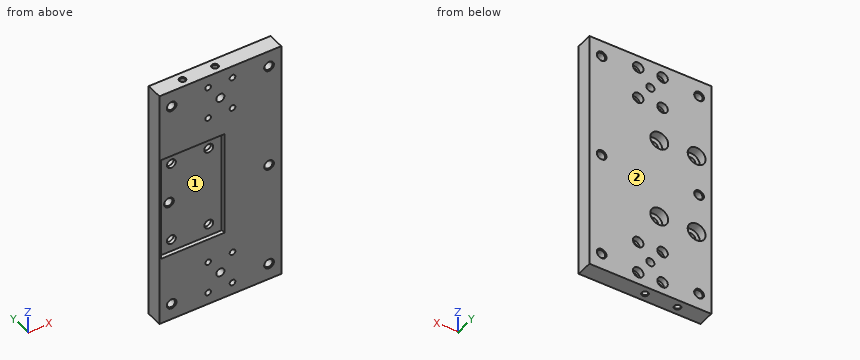
from build123d import *

# Parameters (mm, degrees)
EXTRUDE_1_DEPTH             = 75
EXTRUDE_1_DEPTH_BACK        = 75
SKETCH_1_W                  = 75
SKETCH_1_H                  = 10
SKETCH_2_W                  = 2.5
SKETCH_2_H                  = 10
SKETCH_3_W                  = 2.5
SKETCH_3_H                  = 10
PATTERN_LINEAR_2_COUNT      = 2
PATTERN_LINEAR_2_PITCH      = 23
PATTERN_LINEAR_2_COUNT_DIR2 = 2
PATTERN_LINEAR_2_PITCH_DIR2 = 50
SKETCH_15_W                 = 39
SKETCH_15_H                 = 65
CUT_EXTRUDE_1_DEPTH         = 32.5


with BuildPart() as part:
    # Sketch 1 → Extrude 1 (new, two sides: drawn at the far end of the back side and taken through both)
    with BuildSketch(Plane.XY.offset(-EXTRUDE_1_DEPTH_BACK)):
        with Locations((0, 5)):
            Rectangle(SKETCH_1_W, SKETCH_1_H)
    extrude(amount=EXTRUDE_1_DEPTH + EXTRUDE_1_DEPTH_BACK)

    # Sketch 2 → Cut-Revolve 1 (revolve, cut)
    with BuildSketch(Plane.XY.offset(57.5), mode=Mode.PRIVATE) as cut_revolve_1_sk:
        with Locations((-1.25, 5)):
            Rectangle(SKETCH_2_W, SKETCH_2_H)
    revolve(cut_revolve_1_sk.sketch.rotate(Axis((0, 10, 57.5), (0, -1, 0)), 90), axis=Axis((0, 10, 57.5), (0, -1, 0)), mode=Mode.SUBTRACT)

    # Sketch 3 → Cut-Revolve 2 (revolve, cut)
    with BuildSketch(Plane.XY.offset(-57.5), mode=Mode.PRIVATE) as cut_revolve_2_sk:
        with Locations((-1.25, 5)):
            Rectangle(SKETCH_3_W, SKETCH_3_H)
    revolve(cut_revolve_2_sk.sketch.rotate(Axis((0, 10, -57.5), (0, -1, 0)), 90), axis=Axis((0, 10, -57.5), (0, -1, 0)), mode=Mode.SUBTRACT)

    # Sketch 4 → Cut-Revolve 3 (revolve, cut)
    with BuildSketch(Plane.XY.offset(67.5), mode=Mode.PRIVATE) as cut_revolve_3_sk:
        Polygon((-7.5, 0), (-9.25, 0), (-9.25, 6.5), (-10.75, 6.5), (-10.75, 10), (-7.5, 10), align=None)
    revolve(cut_revolve_3_sk.sketch.rotate(Axis((-7.5, 10, 67.5), (0, -1, 0)), 90), axis=Axis((-7.5, 10, 67.5), (0, -1, 0)), mode=Mode.SUBTRACT)

    # Sketch 6 → Cut-Revolve 4 (revolve, cut)
    with BuildSketch(Plane.XY.offset(-47.5), mode=Mode.PRIVATE) as cut_revolve_4_sk:
        Polygon((7.5, 0), (5.75, 0), (5.75, 6.5), (4.25, 6.5), (4.25, 10), (7.5, 10), align=None)
    revolve(cut_revolve_4_sk.sketch.rotate(Axis((7.5, 10, -47.5), (0, -1, 0)), 90), axis=Axis((7.5, 10, -47.5), (0, -1, 0)), mode=Mode.SUBTRACT)

    # Sketch 7 → Cut-Revolve 5 (revolve, cut)
    with BuildSketch(Plane.XY.offset(-47.5), mode=Mode.PRIVATE) as cut_revolve_5_sk:
        Polygon((-7.5, 0), (-9.25, 0), (-9.25, 6.5), (-10.75, 6.5), (-10.75, 10), (-7.5, 10), align=None)
    revolve(cut_revolve_5_sk.sketch.rotate(Axis((-7.5, 10, -47.5), (0, -1, 0)), 90), axis=Axis((-7.5, 10, -47.5), (0, -1, 0)), mode=Mode.SUBTRACT)

    # Sketch 8 → Cut-Revolve 6 (revolve, cut)
    with BuildSketch(Plane.XY.offset(-67.5), mode=Mode.PRIVATE) as cut_revolve_6_sk:
        Polygon((7.5, 0), (5.75, 0), (5.75, 6.5), (4.25, 6.5), (4.25, 10), (7.5, 10), align=None)
    revolve(cut_revolve_6_sk.sketch.rotate(Axis((7.5, 10, -67.5), (0, -1, 0)), 90), axis=Axis((7.5, 10, -67.5), (0, -1, 0)), mode=Mode.SUBTRACT)

    # Sketch 9 → Cut-Revolve 7 (revolve, cut)
    with BuildSketch(Plane.XY.offset(-67.5), mode=Mode.PRIVATE) as cut_revolve_7_sk:
        Polygon((-7.5, 0), (-9.25, 0), (-9.25, 6.5), (-10.75, 6.5), (-10.75, 10), (-7.5, 10), align=None)
    revolve(cut_revolve_7_sk.sketch.rotate(Axis((-7.5, 10, -67.5), (0, -1, 0)), 90), axis=Axis((-7.5, 10, -67.5), (0, -1, 0)), mode=Mode.SUBTRACT)

    # Sketch 10 → Cut-Revolve 8 (revolve, cut)
    with BuildSketch(Plane.XY.offset(47.5), mode=Mode.PRIVATE) as cut_revolve_8_sk:
        Polygon((7.5, 0), (5.75, 0), (5.75, 6.5), (4.25, 6.5), (4.25, 10), (7.5, 10), align=None)
    revolve(cut_revolve_8_sk.sketch.rotate(Axis((7.5, 10, 47.5), (0, -1, 0)), 90), axis=Axis((7.5, 10, 47.5), (0, -1, 0)), mode=Mode.SUBTRACT)

    # Sketch 11 → Cut-Revolve 9 (revolve, cut)
    with BuildSketch(Plane.XY.offset(47.5), mode=Mode.PRIVATE) as cut_revolve_9_sk:
        Polygon((-7.5, 0), (-9.25, 0), (-9.25, 6.5), (-10.75, 6.5), (-10.75, 10), (-7.5, 10), align=None)
    revolve(cut_revolve_9_sk.sketch.rotate(Axis((-7.5, 10, 47.5), (0, -1, 0)), 90), axis=Axis((-7.5, 10, 47.5), (0, -1, 0)), mode=Mode.SUBTRACT)

    # Sketch 12 → Cut-Revolve 10 (revolve, cut)
    with BuildSketch(Plane.XY.offset(67.5), mode=Mode.PRIVATE) as cut_revolve_10_sk:
        Polygon((7.5, 0), (5.75, 0), (5.75, 6.5), (4.25, 6.5), (4.25, 10), (7.5, 10), align=None)
    revolve(cut_revolve_10_sk.sketch.rotate(Axis((7.5, 10, 67.5), (0, -1, 0)), 90), axis=Axis((7.5, 10, 67.5), (0, -1, 0)), mode=Mode.SUBTRACT)

    # Sketch 13 → Cut-Revolve 11 (revolve, cut)
    with BuildSketch(Plane(origin=(-28.5, 0, 0), x_dir=(0, 0, -1), z_dir=(1, 0, 0)), mode=Mode.PRIVATE) as cut_revolve_11_sk:
        Polygon((-25, 0), (-27.75, 0), (-27.75, 4.6), (-30.5, 4.6), (-30.5, 10), (-25, 10), align=None)
    cut_revolve_11 = revolve(cut_revolve_11_sk.sketch.rotate(Axis((-28.5, 10, 25), (0, -1, 0)), 180), axis=Axis((-28.5, 10, 25), (0, -1, 0)), mode=Mode.SUBTRACT)

    # Pattern Linear 2: Cut-Revolve 11 2 × 2
    with Locations(*[(i * PATTERN_LINEAR_2_PITCH, 0, -j * PATTERN_LINEAR_2_PITCH_DIR2) for i in range(PATTERN_LINEAR_2_COUNT) for j in range(PATTERN_LINEAR_2_COUNT_DIR2) if (i, j) != (0, 0)]):
        add(cut_revolve_11, mode=Mode.SUBTRACT)

    # Sketch 15 → Cut-Extrude 1 (cut)
    with BuildSketch(Plane(origin=(0, 2.5, 0), x_dir=(1, 0, 0), z_dir=(0, 1, 0))):
        with Locations((-17, 0)):
            Rectangle(SKETCH_15_W, SKETCH_15_H)
    extrude(amount=-CUT_EXTRUDE_1_DEPTH, mode=Mode.SUBTRACT)

    # Sketch 16 → Cut-Revolve 12 (revolve, cut)
    with BuildSketch(Plane(origin=(0, 0, 0), x_dir=(0, 0, -1), z_dir=(1, 0, 0)), mode=Mode.PRIVATE) as cut_revolve_12_sk:
        Polygon((-75, 5), (-75, 7), (-74.621, 6.621), (-65.4, 6.621), (-64.464115214, 5), align=None)
    revolve(cut_revolve_12_sk.sketch.rotate(Axis((0, 5, 64.464115214), (0, 0, 1)), 270), axis=Axis((0, 5, 64.464115214), (0, 0, 1)), mode=Mode.SUBTRACT)

    # Sketch 17 → Cut-Revolve 13 (revolve, cut)
    with BuildSketch(Plane(origin=(0, 0, 0), x_dir=(0, 0, -1), z_dir=(1, 0, 0)), mode=Mode.PRIVATE) as cut_revolve_13_sk:
        Polygon((75, 5), (75, 3), (74.621, 3.379), (65.4, 3.379), (64.464115214, 5), align=None)
    revolve(cut_revolve_13_sk.sketch.rotate(Axis((0, 5, -64.464115214), (0, 0, -1)), 180), axis=Axis((0, 5, -64.464115214), (0, 0, -1)), mode=Mode.SUBTRACT)

    # Sketch 18 → Cut-Revolve 14 (revolve, cut)
    with BuildSketch(Plane(origin=(-20, 0, 0), x_dir=(0, 0, -1), z_dir=(1, 0, 0)), mode=Mode.PRIVATE) as cut_revolve_14_sk:
        Polygon((-75, 5), (-75, 7), (-74.621, 6.621), (-65.4, 6.621), (-64.464115214, 5), align=None)
    revolve(cut_revolve_14_sk.sketch.rotate(Axis((-20, 5, 64.464115214), (0, 0, 1)), 270), axis=Axis((-20, 5, 64.464115214), (0, 0, 1)), mode=Mode.SUBTRACT)

    # Sketch 19 → Cut-Revolve 15 (revolve, cut)
    with BuildSketch(Plane(origin=(-20, 0, 0), x_dir=(0, 0, -1), z_dir=(1, 0, 0)), mode=Mode.PRIVATE) as cut_revolve_15_sk:
        Polygon((75, 5), (75, 3), (74.621, 3.379), (65.4, 3.379), (64.464115214, 5), align=None)
    revolve(cut_revolve_15_sk.sketch.rotate(Axis((-20, 5, -64.464115214), (0, 0, -1)), 180), axis=Axis((-20, 5, -64.464115214), (0, 0, -1)), mode=Mode.SUBTRACT)

    # Sketch 20 → Cut-Revolve 16 (revolve, cut)
    with BuildSketch(Plane(origin=(30, 0, 0), x_dir=(0, 0, -1), z_dir=(1, 0, 0)), mode=Mode.PRIVATE) as cut_revolve_16_sk:
        Polygon((-65, 10), (-62, 10), (-62.5415, 9.4585), (-62.5415, 0.5415), (-62, 0), (-65, 0), align=None)
    revolve(cut_revolve_16_sk.sketch.rotate(Axis((30, 0, 65), (0, 1, 0)), 180), axis=Axis((30, 0, 65), (0, 1, 0)), mode=Mode.SUBTRACT)

    # Sketch 21 → Cut-Revolve 17 (revolve, cut)
    with BuildSketch(Plane(origin=(30, 0, 0), x_dir=(0, 0, -1), z_dir=(1, 0, 0)), mode=Mode.PRIVATE) as cut_revolve_17_sk:
        Polygon((65, 10), (68, 10), (67.4585, 9.4585), (67.4585, 0.5415), (68, 0), (65, 0), align=None)
    revolve(cut_revolve_17_sk.sketch.rotate(Axis((30, 0, -65), (0, 1, 0)), 180), axis=Axis((30, 0, -65), (0, 1, 0)), mode=Mode.SUBTRACT)

    # Sketch 22 → Cut-Revolve 18 (revolve, cut)
    with BuildSketch(Plane(origin=(30, 0, 0), x_dir=(0, 0, -1), z_dir=(1, 0, 0)), mode=Mode.PRIVATE) as cut_revolve_18_sk:
        Polygon((0, 10), (3, 10), (2.4585, 9.4585), (2.4585, 0.5415), (3, 0), (0, 0), align=None)
    revolve(cut_revolve_18_sk.sketch.rotate(Axis((30, 0, 0), (0, 1, 0)), 180), axis=Axis((30, 0, 0), (0, 1, 0)), mode=Mode.SUBTRACT)

    # Sketch 23 → Cut-Revolve 19 (revolve, cut)
    with BuildSketch(Plane(origin=(-30, 0, 0), x_dir=(0, 0, -1), z_dir=(1, 0, 0)), mode=Mode.PRIVATE) as cut_revolve_19_sk:
        Polygon((-65, 10), (-62, 10), (-62.5415, 9.4585), (-62.5415, 0.5415), (-62, 0), (-65, 0), align=None)
    revolve(cut_revolve_19_sk.sketch.rotate(Axis((-30, 0, 65), (0, 1, 0)), 180), axis=Axis((-30, 0, 65), (0, 1, 0)), mode=Mode.SUBTRACT)

    # Sketch 24 → Cut-Revolve 20 (revolve, cut)
    with BuildSketch(Plane(origin=(-30, 0, 0), x_dir=(0, 0, -1), z_dir=(1, 0, 0)), mode=Mode.PRIVATE) as cut_revolve_20_sk:
        Polygon((65, 10), (68, 10), (67.4585, 9.4585), (67.4585, 0.5415), (68, 0), (65, 0), align=None)
    revolve(cut_revolve_20_sk.sketch.rotate(Axis((-30, 0, -65), (0, 1, 0)), 180), axis=Axis((-30, 0, -65), (0, 1, 0)), mode=Mode.SUBTRACT)

    # Sketch 25 → Cut-Revolve 21 (revolve, cut)
    with BuildSketch(Plane(origin=(-30, 0, 0), x_dir=(0, 0, -1), z_dir=(1, 0, 0)), mode=Mode.PRIVATE) as cut_revolve_21_sk:
        Polygon((0, 10), (3, 10), (2.4585, 9.4585), (2.4585, 3.0415), (3, 2.5), (0, 2.5), align=None)
    revolve(cut_revolve_21_sk.sketch.rotate(Axis((-30, 2.5, 0), (0, 1, 0)), 180), axis=Axis((-30, 2.5, 0), (0, 1, 0)), mode=Mode.SUBTRACT)


solid = part.part
Design review of the part built by this model. Coordinates are the model's own, in mm. Face numbers are marked on the shaded views. Give positions to 0.01 mm unless a question says otherwise; leave off trailing zeros. Write each loop counter-clockwise with the first axis right and the second up, starting at its lowest first coordinate (ties: lowest second). Pieces come first, ordered by that corner, then holes. Notation, with made-up numbers: M 14.5,59 L 48.5,59 A19 ccw 48.5,86 Z; hole C 66.25,-23.5 d5. An arc over 180 degrees is marked long. Return JSON: item names as keys, results as strings. Group by question number.
Item 1: Take a section at C-C (x = 7.5). Count the separate pieces of the cut face and the enclosed holes in it, plus the area to 3 significant figures.
Item 2: Take a section at B-B (z = -5). Give the boundary of the cut face in (x, y), plus the area to 4 significant figures.
Item 3: The part is to be moulded in two halves that separate along Z. For the marked faces 1 and 2, say which applies: pulls with the +Z half, pulls with the -Z half, needs draft (parallel to the pull), parting line crosses it, or undercut.
Item 4: Clearance check with flat-ended pins moving along their axes: pin 1 Ø5.5 at (x, z) = (-30, -65) entering from +Y; pin 2 Ø1.9 at (x, y) = (-20, 5) entering from -Z; pin 3 Ø6.5 at (x, z) = (-28.5, 25) entering from -Y. State where each tip first meets the part, or that it passes through.
Item 5: Take a section at A-A (x = 30). Give the boundary of the cut face in (y, z).
Item 6: Wall thickness on line 1 along X through (y, z) = (8, -47.5); line 2 along Y through (x, z) = (0, 72.5); line 3 along Z through (x, y) = (-11, 1.5): over which ranges is each line inside the solid? List them lowest first.
Return value:
{
 "1": {"separate pieces": "5", "enclosed holes": "0", "area": "1,320 mm2"},
 "2": {"outline": "M -37.5,0 L -36.5,0 L -36.5,2.5 L 2.5,2.5 L 2.5,0 L 37.5,0 L 37.5,10 L -37.5,10 Z", "area": "652.5 mm2"},
 "3": {"face 1": "undercut", "face 2": "needs draft"},
 "4": {"pin 1": "stops at y = 9.75", "pin 2": "stops at z = -65.01", "pin 3": "stops at y = 2.5"},
 "5": {"outline": "M 0,-75 L 10,-75 L 10,-68 L 9.46,-67.46 L 0.54,-67.46 L 0,-68 Z; M 0,-62 L 0.54,-62.54 L 9.46,-62.54 L 10,-62 L 10,-3 L 9.46,-2.46 L 0.54,-2.46 L 0,-3 Z; M 0,3 L 0.54,2.46 L 9.46,2.46 L 10,3 L 10,62 L 9.46,62.54 L 0.54,62.54 L 0,62 Z; M 0,68 L 0.54,67.46 L 9.46,67.46 L 10,68 L 10,75 L 0,75 Z"},
 "6": {"line 1": "x = -37.5 to -10.75, -4.25 to 4.25, 10.75 to 37.5", "line 2": "y = 0 to 3.38, 6.62 to 10", "line 3": "z = -75 to -32.5, 32.5 to 75"}
}
